For this review, use the dimensioned drawing (mm, ordinates from the lowest corner) and the shaded views. Round coordinates to 2 decimals unless told otherwise and drop trailing zeros. Write each loop counter-clockwise with the first axis right and the second up, starting at its lowest first coordinate (ties: lowest second). Pieces come first, ordered by that corner, then holes. Notation, with made-up numbers: (63, 23.25) -> (103, 23.25) arc R25 cw to (103, 56.25) -> close; hole circle Ø3 at (40, 83). An arc over 180 degrees is marked (long way). Write each question's results on one line, items separated by ' | '. Start each with the question number.
Item 1: Add section B-B (z = 158). State the section outline as (x, y) points (3 decimals), plus the area to 3 significant figures.
Item 2: Add section C-C (y = 2.2). State the section outline as (x, z) points.
Item 3: Add section A-A (x = 99). State the section outline as (y, z) points (3 decimals).
Item 4: Add section D-D (x = 20). State the section outline as (y, z) points (3 decimals), plus the area to 3 significant figures.
Item 5: To check wall thickness, follow line 1 along X through (y, z) = (2.8, 260.5); line 2 along Z through (x, y) = (171.5, 0.9); line 3 along X through (y, z) = (0.5, 330.5). State the ranges of each line that lie inside material, in increasing order.
Item 6: Clearance check with a flat-ended pin moving along its axis: pin 1 (1 mm diameter, centred on y = 2.5, z = 330, fed in from -X). State where the tip first meets the part, or that it passes through.
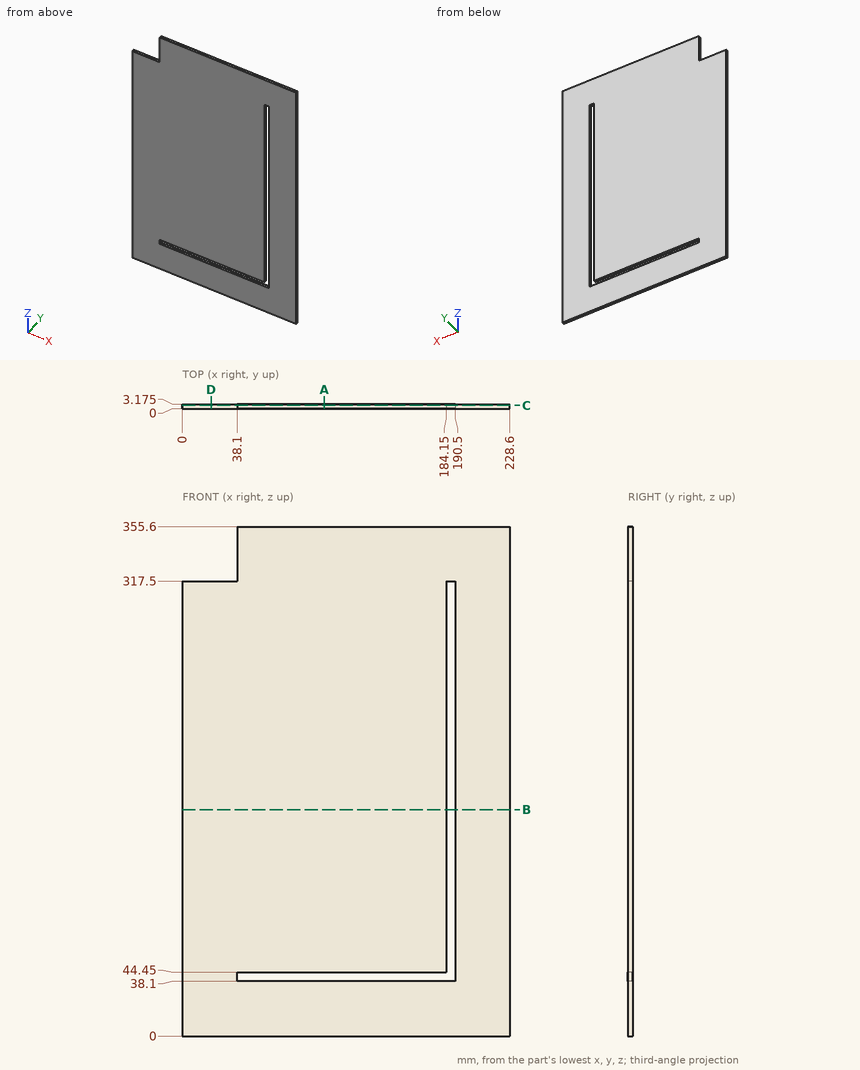
Responses:
1) outline: (0, 0) -> (184.15, 0) -> (184.15, 3.175) -> (0, 3.175) -> close; (190.5, 0) -> (228.6, 0) -> (228.6, 3.175) -> (190.5, 3.175) -> close | area: 706 mm^2
2) outline: (0, 0) -> (228.6, 0) -> (228.6, 355.6) -> (38.1, 355.6) -> (38.1, 317.5) -> (0, 317.5) -> close; hole (38.1, 38.1) -> (190.5, 38.1) -> (190.5, 317.5) -> (184.15, 317.5) -> (184.15, 44.45) -> (38.1, 44.45) -> close
3) outline: (0, 0) -> (3.175, 0) -> (3.175, 38.1) -> (0, 38.1) -> close; (0, 44.45) -> (3.175, 44.45) -> (3.175, 355.6) -> (0, 355.6) -> close
4) outline: (0, 0) -> (3.175, 0) -> (3.175, 317.5) -> (0, 317.5) -> close | area: 1,010 mm^2
5) line 1: x = 0 to 184.15, 190.5 to 228.6 | line 2: z = 0 to 38.1, 44.45 to 355.6 | line 3: x = 38.1 to 228.6
6) pin 1: stops at x = 38.1
